Read the model definition and answer for the solid it produces. Units are mm, in the model's axes. A direction names the side the tool comes from. Round coordinates to 2 decimals unless told otherwise and drop trailing zeros. Write each loop counter-clockwise with the first axis right and the second up, starting at its lowest first coordinate (ties: lowest second). Pieces come first, ordered by that corner, then holes. Notation, with made-up numbers: (48.5, -28.75) - (95.5, -28.75) arc R16 cw to (95.5, -23.75) - close; hole circle Ø6 at (85.5, 13). An arc over 180 degrees is marked (long way). Use one line per item in the form item = value. Start each with the question number.
1) For faces 4 (the face through (43.84, 24.6, 5.59)), 5 (the face through (-42.2, 12.7, 6.6)), 6 (the face through (50.8, 0, 1)), determine the directions among +Z, -Z, +X, -X, +Y, -Y from which every point of the face is accessible in a straight line to the end or side of a thin tool.
2) The part is cut by section A-A, the plane z = 4.75. Give the vertices of the cut face in (x, y).
3) The part is cut by section C-C, the plane y = 23.5. Give the vertices of the cut face in (x, z), plus the area to 3 significant figures.
4) The part is cut by section D-D, the plane y = 5. Give the vertices of the cut face in (x, z).
5) Each of these flat-tipped pins is pushed along its axis until it touches: pin 1 (0.8 mm diameter, centred on x = 11, z = 1.5, fed in from +Y); pin 2 (3 mm diameter, centred on x = -34, y = -1.5, fed in from +Z); pin 3 (1 mm diameter, centred on x = 21.5, y = -23, fed in from -Z); pin 4 (3 mm diameter, centred on y = 21.5, z = 4.5, fed in from +X). Where does it stop, or does it pass through?
6) The part is cut by section B-B, the plane x = -11. Give the vertices of the cut face in (y, z).
7) For a pull along X with two mould halves and no side action, classify faces 1 (the face through (-42, 25, 6.89)), 2 (the face through (38.949, 25, 4)), 3 (the face through (50.036, 37.376, 1.288)) as released by +X, released by -X, zero draft, split by the parting line, or undercut.
8) Consider line 1 along X through (y, z) = (14, 4); line 2 along X through (y, z) = (19.5, 3.5); line 3 along Z through (x, y) = (19.5, 10.5). Determine where each line is inside the solid, lowest interval first. Write a range as from..to.
from build123d import *

# Parameters (mm, degrees)
SKETCH1_W           = 101.6
SKETCH1_H           = 76.2
BOSS_EXTRUDE1_DEPTH = 2.54
SKETCH2_R           = 1.5875
SKETCH2_R_2         = 1.3335
BOSS_EXTRUDE2_DEPTH = 25.4
BOSS_EXTRUDE3_START = 0.254
SKETCH3_R           = 1.5875
BOSS_EXTRUDE3_DEPTH = 0.254
FILLET1_R           = 2.54
BOSS_EXTRUDE4_START = -25.654
SKETCH4_W           = 6.35
SKETCH4_H           = 6.35
BOSS_EXTRUDE4_DEPTH = 25.654
SKETCH5_R           = 2.54
CUT_EXTRUDE1_DEPTH  = 24.13


with BuildPart() as part:
    # Sketch1 → Boss-Extrude1 (new body)
    with BuildSketch(Plane.XY):
        Rectangle(SKETCH1_W, SKETCH1_H)
    extrude(amount=BOSS_EXTRUDE1_DEPTH)

    # Sketch2 → Boss-Extrude2 (add)
    # profile 1 of 2: a face of its own
    with BuildSketch(Plane(origin=(0, 38.1, 0), x_dir=(1, 0, 0), z_dir=(0, 1, 0))):
        with Locations((-42.123995, -3.71475)):
            Circle(SKETCH2_R)
        with Locations((-42.123995, -3.71475)):
            Circle(SKETCH2_R_2, mode=Mode.SUBTRACT)
    # profile 2 of 2: a face of its own
    with BuildSketch(Plane(origin=(0, 38.1, 0), x_dir=(1, 0, 0), z_dir=(0, 1, 0))):
        with Locations((42.123995, -3.71475)):
            Circle(SKETCH2_R)
        with Locations((42.123995, -3.71475)):
            Circle(SKETCH2_R_2, mode=Mode.SUBTRACT)
    extrude(amount=-BOSS_EXTRUDE2_DEPTH)

    # Sketch3 → Boss-Extrude3 (add)
    with BuildSketch(Plane(origin=(0, 38.1, 0), x_dir=(1, 0, 0), z_dir=(0, 1, 0)).offset(BOSS_EXTRUDE3_START)):
        with Locations(Location((-42.123995, -3.71475, 0), (0, 0, 270))):
            Circle(SKETCH3_R)
        with Locations(Location((42.123995, -3.71475, 0), (0, 0, 132.26858443))):
            Circle(SKETCH3_R)
    extrude(amount=-BOSS_EXTRUDE3_DEPTH)

    # Fillet1
    fillet1_edges = [part.edges().sort_by_distance(p)[0] for p in [
        (50.8, -38.1, 1.27),
        (-50.8, -38.1, 1.27),
        (-50.8, 38.1, 1.27),
        (50.8, 38.1, 1.27),
    ]]
    fillet(fillet1_edges, radius=FILLET1_R)

    # Sketch4 → Boss-Extrude4 (add)
    with BuildSketch(Plane(origin=(0, 38.354, 0), x_dir=(1, 0, 0), z_dir=(0, 1, 0)).offset(BOSS_EXTRUDE4_START)):
        with Locations((-42.123995, -3.71475)):
            Rectangle(SKETCH4_W, SKETCH4_H)
        with Locations((42.123995, -3.71475)):
            Rectangle(SKETCH4_W, SKETCH4_H)
    extrude(amount=BOSS_EXTRUDE4_DEPTH)

    # Sketch5 → Cut-Extrude1 (cut)
    with BuildSketch(Plane.XZ.offset(-12.7)):
        with Locations(Location((-42.123995, 3.71475, 0), (0, 0, 270))):
            Circle(SKETCH5_R)
        with Locations(Location((42.123995, 3.71475, 0), (0, 0, 270))):
            Circle(SKETCH5_R)
    extrude(amount=-CUT_EXTRUDE1_DEPTH, mode=Mode.SUBTRACT)


solid = part.part
Geometry results:
q1.face_4 = none
q1.face_5 = +Z, +X, -X, -Y
q1.face_6 = +Z, -Z, +X, +Y, -Y
q2.outline = (-45.3, 12.7) - (-44.44, 12.7) - (-44.44, 36.83) - (-39.8, 36.83) - (-39.8, 12.7) - (-38.95, 12.7) - (-38.95, 38.35) - (-45.3, 38.35) - close; (38.95, 12.7) - (39.8, 12.7) - (39.8, 36.83) - (44.44, 36.83) - (44.44, 12.7) - (45.3, 12.7) - (45.3, 38.35) - (38.95, 38.35) - close
q3.outline = (-50.8, 0) - (50.8, 0) - (50.8, 2.54) - (45.3, 2.54) - (45.3, 6.89) - (38.95, 6.89) - (38.95, 2.54) - (-38.95, 2.54) - (-38.95, 6.89) - (-45.3, 6.89) - (-45.3, 2.54) - (-50.8, 2.54) - close; hole circle Ø5.08 at (-42.12, 3.71); hole circle Ø5.08 at (42.12, 3.71)
q3.area = 273 mm2
q4.outline = (-50.8, 0) - (50.8, 0) - (50.8, 2.54) - (-50.8, 2.54) - close
q5.pin_1 = 38.1
q5.pin_2 = 2.54
q5.pin_3 = 0
q5.pin_4 = 45.3
q6.outline = (-38.1, 0) - (38.1, 0) - (38.1, 2.54) - (-38.1, 2.54) - close
q7.face_1 = zero draft
q7.face_2 = undercut
q7.face_3 = released by +X
q8.line_1 = -45.3..-44.65, -39.6..-38.95, 38.95..39.6, 44.65..45.3
q8.line_2 = -45.3..-44.65, -39.59..-38.95, 38.95..39.59, 44.65..45.3
q8.line_3 = 0..2.54
